Here's how the part is built. I have some questions about the finished solid (model axes, mm). Face numbers are marked on the shaded views. A direction names the side the tool comes from. Give positions to 0.01 mm unless a question says otherwise; leave off trailing zeros. Write each loop counter-clockwise with the first axis right and the second up, starting at its lowest first coordinate (ties: lowest second). Pieces come first, ordered by that corner, then holes. Notation, with made-up numbers: (82.25, 55.25) -> (137.25, 55.25) arc R18 ccw to (137.25, 88.25) -> close; hole circle Ø5 at (-15, 67). An arc over 180 degrees is marked (long way). Return JSON: item names as keys, results as strings.
from build123d import *

# Parameters (mm, degrees)
F0_W     = 103.285306
F0_H     = 12.7
F1_DEPTH = 50.8
F0_H_2   = 25.4
F2_DEPTH = 20
F3_R     = 5
F4_DEPTH = 25


with BuildPart() as f1:
    # F0 (on Top) → F1 (new body)
    with BuildSketch(Plane.XY):
        with Locations((0, 19.05)):
            Rectangle(F0_W, F0_H)
        with Locations((0, -19.05)):
            Rectangle(F0_W, F0_H)
    extrude(amount=F1_DEPTH)

    # F0 (on Top) → F2 (join)
    with BuildSketch(Plane.XY):
        Rectangle(F0_W, F0_H_2)
    extrude(amount=F2_DEPTH)

    # F3 (on face) → F4 (join)
    with BuildSketch(Plane.XY):
        Circle(F3_R)
    extrude(amount=-F4_DEPTH)


solid = f1.part
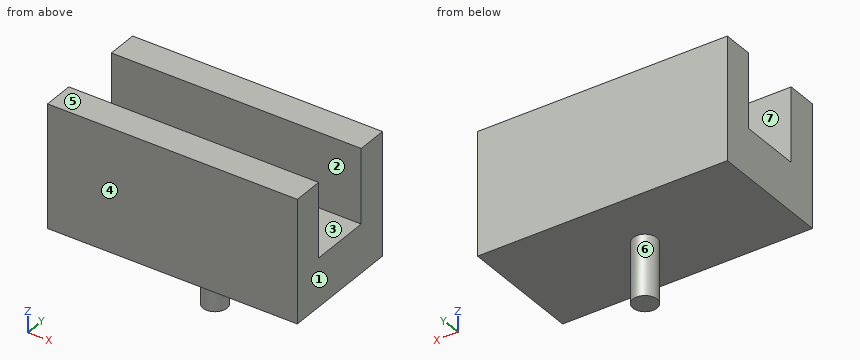
1. If I drill on line 1 (Y direction, x = -8, z = 36); line 2 (Z direction, x = 44, y = 21.5); line 3 (Z direction, x = 11.5, y = 12.5), over which ranges is the centre line in solid material (lowest first)? Write a range as [from, to].
Taken from the geometry:
{"line 1": "y = [-25.4, -12.7], [12.7, 25.4]", "line 2": "z = [0, 50.8]", "line 3": "z = [0, 20]"}
2. Suppose I cut it at B-B, the plane x = 0. List the corners of the cut face in (y, z) for me.
Taken from the geometry:
{"outline": "(-25.4, 0) -> (-5, 0) -> (-5, -25) -> (5, -25) -> (5, 0) -> (25.4, 0) -> (25.4, 50.8) -> (12.7, 50.8) -> (12.7, 20) -> (-12.7, 20) -> (-12.7, 50.8) -> (-25.4, 50.8) -> close"}
3. For pin 1 Ø1.5 at (x, y) = (-22.5, -15) entering from -Z; pin 2 Ø7.5 at (x, y) = (-21, 1.5) entering from +Z; pin 3 Ø1 at (x, z) = (-2, -16) entering from -Y, each with a flat end and sliding along its axis, tell me the tip position at first contact or that it passes through.
Taken from the geometry:
{"pin 1": "stops at z = 0", "pin 2": "stops at z = 20", "pin 3": "stops at y = -4.77"}
4. If we mould it in two halves opening along Y, with no side actions, what happens to the marked faces 1, 2, 3 and 4? For each: released by +Y, released by -Y, zero draft, split by the parting line, or undercut.
Taken from the geometry:
{"face 1": "zero draft", "face 2": "undercut", "face 3": "undercut", "face 4": "released by -Y"}
5. Which directions (+Z, -Z, +X, -X, +Y, -Y) give clear straight access to the entire face, cutting with the end or side of a thin tool? Please do the marked faces 5, 6 and 7.
Taken from the geometry:
{"face 5": "+Z, +X, -X, +Y, -Y", "face 6": "-Z", "face 7": "+Z, +X, -X"}
6. Suppose I cut it at A-A, the plane y = 0. List the corners of the cut face in (x, z) for me, and give its area (3 significant figures).
Taken from the geometry:
{"outline": "(-51.64, 0) -> (-5, 0) -> (-5, -25) -> (5, -25) -> (5, 0) -> (51.64, 0) -> (51.64, 20) -> (-51.64, 20) -> close", "area": "2,320 mm²"}
7. Suppose I cut it at C-C, the plane x = -27.5. List the corners of the cut face in (y, z) for me.
Taken from the geometry:
{"outline": "(-25.4, 0) -> (25.4, 0) -> (25.4, 50.8) -> (12.7, 50.8) -> (12.7, 20) -> (-12.7, 20) -> (-12.7, 50.8) -> (-25.4, 50.8) -> close"}
8. Suppose I cut it at D-D, the plane y = -8. List the corners of the cut face in (x, z) for me.
Taken from the geometry:
{"outline": "(-51.64, 0) -> (51.64, 0) -> (51.64, 20) -> (-51.64, 20) -> close"}
